Autodesk Inventor part; units mm, degrees
ref_plane "YZ Plane" through (0, 0, 0) normal (1, 0, 0) x (0, 1, 0)
ref_plane "XZ Plane" through (0, 0, 0) normal (0, 1, 0) x (-1, 0, 0)
ref_plane "XY Plane" through (0, 0, 0) normal (0, 0, 1) x (1, 0, 0)
sketch "Sketch1" plane through (0, 0, 0) normal (0, 0, 1) x (1, 0, 0)
  line L0 (0, 0) -> (29, 0)
  line L1 (29, 0) -> (43.462, 119.715)
  line L2 (43.462, 119.715) -> (45.3715, 121.8246)
  line L3 (45.3715, 121.8246) -> (49.5, 156)
  line L4 (49.5, 156) -> (0, 156) construction
  line L5 (0, 156) -> (0, 0) construction
  line L6 (0, 0) -> (0, 2)
  line L7 (0, 2) -> (27.2271, 2)
  line L8 (27.2271, 2) -> (41.5527, 120.5859)
  line L9 (41.5527, 120.5859) -> (43.4622, 122.6955)
  line L10 (43.4622, 122.6955) -> (47.4855, 156)
  line L11 (49.5, 156) -> (47.4855, 156)
  dimension "d1" = 29
  dimension "d2" = 49.5
  dimension "d3" = 156
  dimension "d24" = 2
  dimension "d25" = 2
  dimension "d26" = 2
  dimension "d27" = 2
revolve "Revolution1" add sketch "Sketch1" angle 360 about axis through (0, 156, 0) along (0, -1, 0)
equation "\"d24\" = PopcornCup_Thickness"
equation "\"d25\" = PopcornCup_Thickness"
equation "\"d26\" = PopcornCup_Thickness"
equation "\"d27\" = PopcornCup_Thickness"
equation "\"PopcornCup_Thickness\" = 2"
equation "\"PopcornCup_Base_DiameterMax\" = 58"
properties part number "PopcornCup" material "Polycarbonate, Clear"
Build history of the part. All positions in model axes, mm. Give positions to 0.01 mm unless a question says otherwise; leave off trailing zeros. Loops run counter-clockwise (first coordinate to the right, second up) from the corner with the lowest first, then second, coordinate; pieces in that order, holes last. Notation, with made-up numbers: (67.5, 86) - (122.5, 86) arc R16 cw to (122.5, 92) - close; hole circle Ø8 at (2.25, 59). An arc over 180 degrees is marked (long way). Write item = value, one per line. Start each with the question number.
1) Probe probe 1 along X at (y, z) = (90, 32.5); probe 2 along Z at (x, y) = (-33.5, 107); probe 3 along X at (y, z) = (116, 28). List the from-to ranges inside material, lowest first. Write a range as from..to.
2) Band-saw the part on B-B on z = 0. Give the cut face in (x, y) (1 decimal).
3) Band-saw the part on A-A on x = 0. Give the cut face in (y, z) (1 decimal), plus the area to 3 significant figures.
4) Band-saw the part on C-C on y = 39. Give the cut face in (x, z), plus the area to 3 significant figures.
5) Drop flat-ended pins along their axis: pin 1 Ø12 at (x, y) = (31, 28.5) entering from +Z; pin 2 Ø2 at (y, z) = (115.5, -32) entering from +X; pin 3 Ø10 at (x, y) = (-27.5, 132) entering from +Z; pin 4 Ø6 at (x, z) = (-38, -39) entering from -Y. Give the stop position or say it passes through.
6) Band-saw the part on D-D on y = 139. Give the cut face in (x, z).
7) Pull direction X, two halves, no side cores. Call faces 1 (the conical face through (-5.87, 135.88, -44.67)), 2 (the conical face through (-7.88, 60.7, 35.47)), 3 (the flat face through (0, 2, 0)), 4 (the flat face through (0, 0, 0)): +X half, -X half, draft (parallel to the pull), parting line (faces both ways), or undercut.
Final values:
q1.probe_1 = -23.1..-19.42, 19.42..23.1
q1.probe_2 = -25.21..-21.7, 21.7..25.21
q1.probe_3 = -32.65..-29.95, 29.95..32.65
q2.outline = (-49.5, 156) - (-45.4, 121.8) - (-43.5, 119.7) - (-29, 0) - (29, 0) - (43.5, 119.7) - (45.4, 121.8) - (49.5, 156) - (47.5, 156) - (43.5, 122.7) - (41.6, 120.6) - (27.2, 2) - (-27.2, 2) - (-41.6, 120.6) - (-43.5, 122.7) - (-47.5, 156) - close
q3.outline = (0, -29) - (119.7, -43.5) - (121.8, -45.4) - (156, -49.5) - (156, -47.5) - (122.7, -43.5) - (120.6, -41.6) - (2, -27.2) - (2, 27.2) - (120.6, 41.6) - (122.7, 43.5) - (156, 47.5) - (156, 49.5) - (121.8, 45.4) - (119.7, 43.5) - (0, 29) - close
q3.area = 740 mm²
q4.outline = circle Ø67.42 at (0, 0); hole circle Ø63.39 at (0, 0)
q4.area = 414 mm²
q5.pin_1 = 20.77
q5.pin_2 = 29.75
q5.pin_3 = 40.89
q5.pin_4 = through
q6.outline = circle Ø94.89 at (0, 0); hole circle Ø90.86 at (0, 0)
q7.face_1 = undercut
q7.face_2 = parting line
q7.face_3 = undercut
q7.face_4 = draft
